Geometry: final body of the model. Coordinates: model frame, mm. Face numbers are marked on the shaded views. Give positions to 0.01 mm unless a question says otherwise; leave off trailing zeros. Order: outer loops, then holes, each group sorted by start corner. A loop starts at its lowest first (then second) coordinate and runs counter-clockwise, first axis right, second up. Notation, with made-up numbers: M 43,28 L 91,28 A15 ccw 91,49 Z; hole C 43.25,41 d1. An arc over 180 degrees is marked long. Use CSV: the item, a comma, the result in double quotes.
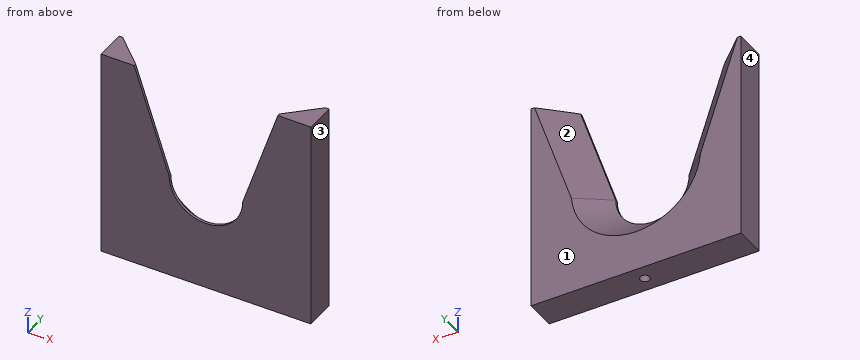
```python
from build123d import *

# Parameters (mm, degrees)
BOSS_EXTRUDE1_DEPTH           = 11.1125
CHAMFER1_SIZE                 = 10.16
TAP_DRILL_FOR_8_32_TAP1_D     = 3.4544
TAP_DRILL_FOR_8_32_TAP1_DEPTH = 15.24
TAP_DRILL_FOR_8_32_TAP1_TIP   = 1.037806461


with BuildPart() as part:
    # Sketch1 → Boss-Extrude1 (new body)
    with BuildSketch(Plane(origin=(0, 0, 0), x_dir=(1, 0, 0), z_dir=(0, 1, 0))):
        with BuildLine():
            Line((-26.083081673, -38.1), (-13.335, 0))
            ThreePointArc((-13.335, 0), (0, 13.335), (13.335, 0))
            Line((13.335, 0), (26.083081673, -38.1))
            Line((26.083081673, -38.1), (38.1, -38.1))
            Line((38.1, -38.1), (38.1, 38.1))
            Line((38.1, 38.1), (-38.1, 38.1))
            Line((-38.1, 38.1), (-38.1, -38.1))
            Line((-38.1, -38.1), (-26.083081673, -38.1))
        make_face()
    extrude(amount=BOSS_EXTRUDE1_DEPTH)

    # Chamfer1
    chamfer1_edges = [part.edges().sort_by_distance(p)[0] for p in [
        (19.709040837, 11.1125, 19.05),
        (-19.709040837, 11.1125, 19.05),
        (0, 11.1125, -13.335),
    ]]
    chamfer(chamfer1_edges, length=CHAMFER1_SIZE)

    # Tap Drill for #8-32 Tap1
    with Locations(Plane(origin=(0, 5.55625, -38.1), x_dir=(-1, 0, 0), z_dir=(0, 0, -1))):
        with Locations((0, 0)):
            Hole(TAP_DRILL_FOR_8_32_TAP1_D / 2, depth=TAP_DRILL_FOR_8_32_TAP1_DEPTH)
            with Locations((0, 0, -(TAP_DRILL_FOR_8_32_TAP1_DEPTH + TAP_DRILL_FOR_8_32_TAP1_TIP / 2))):  # 118° drill point
                Cone(0, TAP_DRILL_FOR_8_32_TAP1_D / 2, TAP_DRILL_FOR_8_32_TAP1_TIP, mode=Mode.SUBTRACT)


solid = part.part
```
1. Section D-D, the plane x = -32. Return the cut outline in (y, z).
Answer:
outline,"M 0,-38.1 L 11.11,-38.1 L 11.11,23.76 L 6.56,38.1 L 0,38.1 Z"
2. Section A-A, the plane z = 24. Return the cut outline in (x, y), plus the area to 3 significant figures.
Answer:
outline,"M -38.1,0 L -21.37,0 L -21.37,0.95 L -32.08,11.11 L -38.1,11.11 Z; M 21.37,0 L 38.1,0 L 38.1,11.11 L 32.08,11.11 L 21.37,0.95 Z"
area,"263 mm2"
3. Line query: line 1 (Y direction, x = 0, z = -33.75); line 2 (X direction, y = 4.75, z = -12); line 3 (X direction, y = 7, z = 34). Output: solid intervals per line, ascending.
Answer:
line 1,"0 to 3.83, 7.28 to 11.11"
line 2,"-38.1 to -12.23, 12.23 to 38.1"
line 3,"-38.1 to -31.09, 31.09 to 38.1"
4. Pull-direction query (X, two-part tool) for the marked faces 1, 2, 3 and 4; classes: +X half, -X half, draft (parallel to the pull), parting line (faces both ways), or undercut.
Answer:
face 1,"draft"
face 2,"undercut"
face 3,"+X half"
face 4,"-X half"
5. Section C-C, the plane z = 32.5. Return the cut outline in (x, y).
Answer:
outline,"M -38.1,0 L -24.21,0 L -24.21,0.95 L -34.92,11.11 L -38.1,11.11 Z; M 24.21,0 L 38.1,0 L 38.1,11.11 L 34.92,11.11 L 24.21,0.95 Z"
6. Pin query (flat end, axial travel): pin 1 Ø5 at (x, z) = (-10, 5) entering from +Y; pin 2 Ø5.5 at (x, y) = (0, 5.56) entering from +Z. Return the tip coordinate at first contact, or that it passes through.
Answer:
pin 1,"through"
pin 2,"z = -15.19"
7. Section B-B, the plane y = 10. Return the cut outline in (x, z) (1 decimal), plus the area to 3 significant figures.
Answer:
outline,"M -38.1,-38.1 L 38.1,-38.1 L 38.1,38.1 L 35.6,38.1 L 22.3,-1.7 A22.4 cw -22.3,-1.7 L -35.6,38.1 L -38.1,38.1 Z"
area,"2,790 mm2"
